```python
from build123d import *

# Parameters (mm, degrees)
BOSS_EXTRUDE1_START = -195
SKETCH1_R           = 127.5
BOSS_EXTRUDE1_DEPTH = 6
BOSS_EXTRUDE2_START = -65
SKETCH2_R           = 4
BOSS_EXTRUDE2_DEPTH = 21


with BuildPart() as part:
    # Sketch1 → Boss-Extrude1 (new body)
    with BuildSketch(Plane(origin=(0, 0, 0), x_dir=(1, 0, 0), z_dir=(0, 1, 0)).offset(BOSS_EXTRUDE1_START)):
        with Locations(Location((0, 0, 0), (0, 0, 270))):
            Circle(SKETCH1_R)
    extrude(amount=BOSS_EXTRUDE1_DEPTH)

    # Sketch2 → Boss-Extrude2 (add, symmetric)
    with BuildSketch(Plane.XY.offset(BOSS_EXTRUDE2_START)):
        with BuildLine():
            Line((-15, 0), (-15, -189))
            Line((-15, -189), (15, -189))
            Line((15, -189), (15, 0))
            ThreePointArc((15, 0), (0, 15), (-15, 0))
        make_face()
        with Locations(Location((0, 0, 0), (0, 0, 180))):
            Circle(SKETCH2_R, mode=Mode.SUBTRACT)
        with Locations(Location((0, -171, 0), (0, 0, 180))):
            Circle(SKETCH2_R, mode=Mode.SUBTRACT)
    extrude(amount=BOSS_EXTRUDE2_DEPTH, both=True)


solid = part.part
```
Work out the finished part from the listing and answer in its coordinate system (mm). A direction names the side the tool comes from. Coordinates: 2 decimals unless noted, no trailing zeros. Loops run counter-clockwise (first coordinate to the right, second up) from the corner with the lowest first, then second, coordinate; pieces in that order, holes last. Notation, with made-up numbers: (26.25, 28) -> (58.25, 28) arc R31 cw to (58.25, 58) -> close; hole circle Ø1 at (-19.75, 64.25). An arc over 180 degrees is marked (long way). Answer as CSV lines item,"result".
Q1. The part is cut by section A-A on x = 0. Write down the section's boundary in (y, z).
Findings:
outline,"(-195, -127.5) -> (-189, -127.5) -> (-189, -86) -> (-175, -86) -> (-175, -44) -> (-189, -44) -> (-189, 127.5) -> (-195, 127.5) -> close; (-167, -86) -> (-4, -86) -> (-4, -44) -> (-167, -44) -> close; (4, -86) -> (15, -86) -> (15, -44) -> (4, -44) -> close"
Q2. A tool of negligible diameter and unlimited length cuts with its end or side. For faces 1 (the face through (15, -96, -65)), 2 (the face through (0, 15, -65)), 3 (the face through (0, -86, -86)), 4 (the face through (0, -86, -44)), from which of +Z, -Z, +X, -X, +Y, -Y can it reach the whole face along a straight path? Write none if from no direction.
Findings:
face 1,"+Z, -Z, +X, +Y"
face 2,"+Z, -Z, +Y"
face 3,"-Z, +X, -X, +Y"
face 4,"+Z, +X, -X, +Y"
Q3. For a pull along X with two mould halves and no side action, classify faces 5 (the face through (0.521, -174.966, -65.294)), 6 (the face through (-15, -93, -65)), 7 (the face through (2, -195, -2)) as +X half, -X half, draft (parallel to the pull), parting line (faces both ways), or undercut.
Findings:
face 5,"undercut"
face 6,"-X half"
face 7,"draft"
Q4. The part is cut by section C-C on y = -52.5. Write down the section's boundary in (x, z).
Findings:
outline,"(-15, -86) -> (15, -86) -> (15, -44) -> (-15, -44) -> close"
Q5. Each of these flat-tipped pins is pushed along its axis until it touches: pin 1 (10 mm diameter, centred on x = -4.5, y = -86.5, fed in from +Z); pin 2 (10.5 mm diameter, centred on x = 0, y = 0, fed in from -Z). Where does it stop, or does it pass through?
Findings:
pin 1,"stops at z = -44"
pin 2,"stops at z = -86"
Q6. The part is cut by section D-D on z = -52. Write down the section's boundary in (x, y).
Findings:
outline,"(-116.41, -195) -> (116.41, -195) -> (116.41, -189) -> (15, -189) -> (15, 0) arc R15 ccw to (-15, 0) -> (-15, -189) -> (-116.41, -189) -> close; hole circle Ø8 at (0, -171); hole circle Ø8 at (0, 0)"
Q7. The part is cut by section B-B on z = 0. Write down the section's boundary in (x, y).
Findings:
outline,"(-127.5, -195) -> (127.5, -195) -> (127.5, -189) -> (-127.5, -189) -> close"
Q8. Find the intervals of material crossed by probe 1 along Y at (x, z) = (0, -53); probe 2 along X at (y, z) = (-171, -61); probe 3 along Y at (x, z) = (-3.5, -57.5), in increasing order.
Findings:
probe 1,"y = -195 to -175, -167 to -4, 4 to 15"
probe 2,"x = -15 to -4, 4 to 15"
probe 3,"y = -195 to -172.94, -169.06 to -1.94, 1.94 to 14.59"
